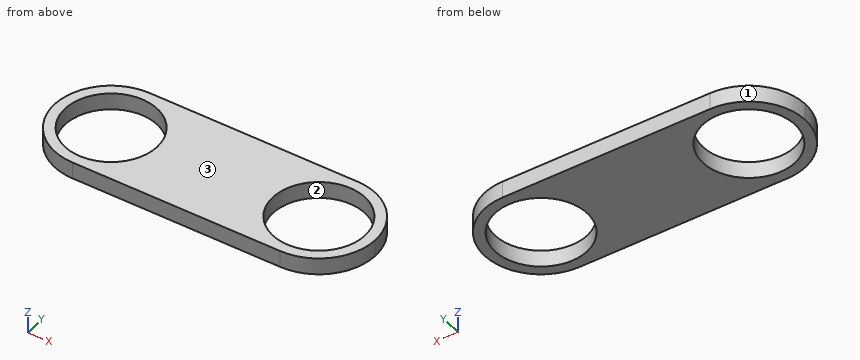
Solid Edge part; units mm, degrees
sketch "Sketch1" plane through (0, 0, 0) normal (0, 0, 1) x (1, 0, 0)
  circle A0 centre (-25, 0) radius 11
  line L0 (38.5, -13.5) -> (-38.5, -13.5)
  line L1 (-38.5, -13.5) -> (-38.5, 13.5)
  line L2 (-38.5, 13.5) -> (38.5, 13.5)
  line L3 (38.5, 13.5) -> (38.5, -13.5)
  circle A1 centre (25, 0) radius 11
extrude "Protrusion1" add sketch "Sketch1" along normal blind 4
fillet "Round_1" radius 13.5 4 edges at (-38.5, -13.5, 2) (-38.5, 13.5, 2) (38.5, 13.5, 2) (38.5, -13.5, 2)
Can you work these out from the model? Positions are in its coordinate system, mm. Face numbers are marked on the shaded views. Round coordinates to 2 decimals unless told otherwise and drop trailing zeros. Loops run counter-clockwise (first coordinate to the right, second up) from the corner with the lowest first, then second, coordinate; pieces in that order, holes last. Notation, with made-up numbers: (13.25, 49.25) - (59.25, 49.25) arc R26 cw to (59.25, 66.25) - close; hole circle Ø4 at (28.25, 40.5). An arc over 180 degrees is marked (long way). Answer in a Markdown table with one row per item. Add a question column.
Q1. We'd pull the mould along X, two halves only. Please class the marked faces 1, 2 and 3: pulls with the +X half, pulls with the -X half, needs draft (parallel to the pull), parting line crosses it, or undercut.
Q2. I need wall thicknesses on L1, parallel to X at y = -4, z = 0.8; L2, parallel to Y at x = 25, z = 3; L3, parallel to X at y = 3.5, z = 2.6. Which ranges of each line are inside material? Lowest first, please.
Q3. I want a section at B-B on y = 9.5. List the corners of the cut face in (x, z) for me, and give its area (3 significant figures).
Q4. For pin 1 Ø2 at (x, y) = (4.5, -8.5) entering from -Z, with a flat end and sliding along its axis, tell me the tip position at first contact or that it passes through.
Q5. I want a section at D-D on y = -7.5. List the corners of the cut face in (x, z) for me, and give its area (3 significant figures).
Q6. I want a section at C-C on z = 1. Count the separate pieces of the cut face and the enclosed holes in it, and give its area (3 significant figures).
Q7. I want a section at A-A on x = -17.5. List the corners of the cut face in (y, z) for me.
A:
| question | item | result |
|---|---|---|
| 1 | face 1 | pulls with the -X half |
| 1 | face 2 | undercut |
| 1 | face 3 | needs draft |
| 2 | L1 | -37.89 to -35.25, -14.75 to 14.75, 35.25 to 37.89 |
| 2 | L2 | -13.5 to -11, 11 to 13.5 |
| 2 | L3 | -38.04 to -35.43, -14.57 to 14.57, 35.43 to 38.04 |
| 3 | outline | (-34.59, 0) - (-30.55, 0) - (-30.55, 4) - (-34.59, 4) - close; (-19.45, 0) - (19.45, 0) - (19.45, 4) - (-19.45, 4) - close; (30.55, 0) - (34.59, 0) - (34.59, 4) - (30.55, 4) - close |
| 3 | area | 188 mm^2 |
| 4 | pin 1 | z = 0 |
| 5 | outline | (-36.23, 0) - (-33.05, 0) - (-33.05, 4) - (-36.23, 4) - close; (-16.95, 0) - (16.95, 0) - (16.95, 4) - (-16.95, 4) - close; (33.05, 0) - (36.23, 0) - (36.23, 4) - (33.05, 4) - close |
| 5 | area | 161 mm^2 |
| 6 | separate pieces | 1 |
| 6 | enclosed holes | 2 |
| 6 | area | 1,160 mm^2 |
| 7 | outline | (-13.5, 0) - (-8.05, 0) - (-8.05, 4) - (-13.5, 4) - close; (8.05, 0) - (13.5, 0) - (13.5, 4) - (8.05, 4) - close |
